Check sheet for the modelled part. Datum: model origin and axes. Units: mm. Face numbers are marked on the shaded views. A direction names the side the tool comes from. Round coordinates to 2 decimals unless told otherwise and drop trailing zeros. Write each loop counter-clockwise with the first axis right and the second up, starting at its lowest first coordinate (ties: lowest second). Pieces come first, ordered by that corner, then holes. Notation, with made-up numbers: (66, -21.75) -> (82, -21.75) arc R23 cw to (82, 16.25) -> close; hole circle Ø11 at (-5, 32). An arc over 180 degrees is marked (long way). One line per item, written item: value. Start each with the question number.
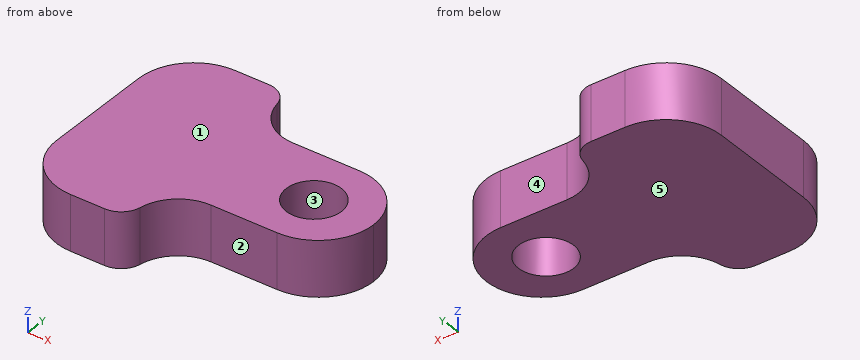
```python
from build123d import *

# Parameters (mm, degrees)
F0_R     = 3.175
F1_DEPTH = 6.35
F2_R     = 5.08
F3_R     = 2.54


with BuildPart() as f1:
    # F0 (on Top) → F1 (new body)
    with BuildSketch(Plane.XY):
        with BuildLine():
            Line((6.35, 6.35), (6.35, 12.7))
            Line((6.35, 12.7), (0, 12.7))
            ThreePointArc((0, 12.7), (-4.490128, 10.840128), (-6.35, 6.35))
            Line((-6.35, 6.35), (-6.35, -6.35))
            ThreePointArc((-6.35, -6.35), (-4.490128, -10.840128), (0, -12.7))
            Line((0, -12.7), (6.35, -12.7))
            Line((6.35, -12.7), (6.35, -6.35))
            Line((6.35, -6.35), (12.7, -6.35))
            Line((12.7, -6.35), (19.05, -6.35))
            ThreePointArc((19.05, -6.35), (23.540128, -4.490128), (25.4, 0))
            ThreePointArc((25.4, 0), (23.540128, 4.490128), (19.05, 6.35))
            Line((19.05, 6.35), (6.35, 6.35))
        make_face()
        with Locations((18.548694, 0)):
            Circle(F0_R, mode=Mode.SUBTRACT)
    extrude(amount=F1_DEPTH)

    # F2
    f2_edges = [f1.edges().sort_by_distance(p)[0] for p in [
        (6.35, -6.35, 3.175),
        (6.35, 6.35, 3.175),
    ]]
    fillet(f2_edges, radius=F2_R)

    # F3
    f3_edges = [f1.edges().sort_by_distance(p)[0] for p in [
        (6.35, 12.7, 3.175),
        (6.35, -12.7, 3.175),
    ]]
    fillet(f3_edges, radius=F3_R)


solid = f1.part
```
1. Depth check by flat-ended pin: pin 1 Ø3 at (x, z) = (16, 4.5) entering from +Y; pin 2 Ø1 at (x, z) = (21, 3.5) entering from +Y; pin 3 Ø1.9 at (x, z) = (14.5, 2.5) entering from -Y; pin 4 Ø4 at (x, y) = (9, -4) entering from -Z. Enter the tip coordinate at first touch or a pass-through.
2. Access from +Z, -Z, +X, -X, +Y, -Y to the whole of each face (thin tool, end or side, straight path). Record for the marked faces 1 and 2.
3. Cross-section at C-C (y = -9.5). Record the cut outline in (x, z), plus the area to 3 significant figures.
4. Cross-section at A-A (y = 1.75). Record the cut outline in (x, z).
5. Cross-section at B-B (y = 7). Record the cut outline in (x, z).
6. Release check for a two-part mould opening along Y. For the marked faces 3, 4 and 5 record: +Y half, -Y half, draft (parallel to the pull), parting line (faces both ways), or undercut.
7. Material ranges on probe 1 along Y at (x, z) = (20, 5.25); probe 2 along Y at (x, z) = (16, 2.75); probe 3 along Y at (x, z) = (13.5, 3), recorded low to high.
Working result:
1. pin 1: stops at y = 6.35
1. pin 2: stops at y = 6.18
1. pin 3: stops at y = -6.35
1. pin 4: stops at z = 0
2. face 1: +Z, +X, -X, +Y, -Y
2. face 2: +Z, -Z, +X, -Y
3. outline: (-5.51, 0) -> (6.73, 0) -> (6.73, 6.35) -> (-5.51, 6.35) -> close
3. area: 77.8 mm^2
4. outline: (-6.35, 0) -> (15.9, 0) -> (15.9, 6.35) -> (-6.35, 6.35) -> close; (21.2, 0) -> (25.15, 0) -> (25.15, 6.35) -> (21.2, 6.35) -> close
5. outline: (-6.32, 0) -> (8.94, 0) -> (8.94, 6.35) -> (-6.32, 6.35) -> close
6. face 3: undercut
6. face 4: +Y half
6. face 5: draft
7. probe 1: y = -6.28 to -2.82, 2.82 to 6.28
7. probe 2: y = -6.35 to -1.89, 1.89 to 6.35
7. probe 3: y = -6.35 to 6.35
